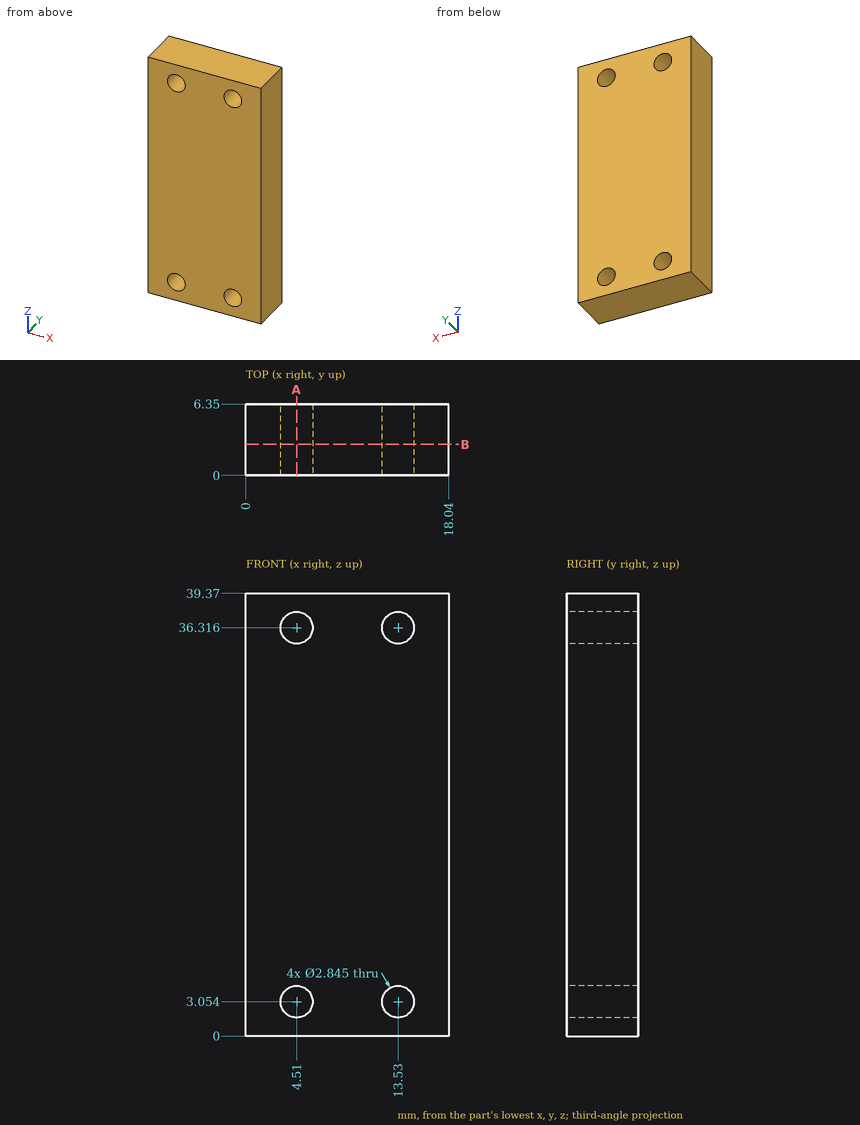
Study the drawing (mm; zero at the part's minimum x, y, z) and answer. Round coordinates to 2 decimals unless told otherwise and drop trailing zeros. Write each loop counter-clockwise with the first axis right and the second up, starting at its lowest first coordinate (ties: lowest second). Pieces come first, ordered by that corner, then holes. Notation, with made-up numbers: (32, 5.5) -> (38, 5.5) arc R17 ccw to (38, 17.5) -> close; hole circle Ø3 at (72.25, 48.5). An arc over 180 degrees is marked (long way). Write item = value, one per line.
1) Section B-B on y = 2.75 is taken. Write down the section's boundary in (x, z) (1 decimal), plus the area to 3 significant figures.
Check values:
outline = (0, 0) -> (18, 0) -> (18, 39.4) -> (0, 39.4) -> close; hole circle Ø2.8 at (4.5, 3.1); hole circle Ø2.8 at (4.5, 36.3); hole circle Ø2.8 at (13.5, 3.1); hole circle Ø2.8 at (13.5, 36.3)
area = 685 mm²
2) Section A-A on x = 4.51 is taken. Write down the section's boundary in (y, z).
Check values:
outline = (0, 0) -> (6.35, 0) -> (6.35, 1.63) -> (0, 1.63) -> close; (0, 4.48) -> (6.35, 4.48) -> (6.35, 34.89) -> (0, 34.89) -> close; (0, 37.74) -> (6.35, 37.74) -> (6.35, 39.37) -> (0, 39.37) -> close
3) Given pin 1 (1.7 mm diameter, centred on x = 13.53, z = 36.32, fed in from -Y), flat-ended and moving along its own axis, determine where the tip first touches the part or whether it passes through.
Check values:
pin_1 = through
4) Straight lines are drawn through the part: line 1 along Z through (x, y) = (13.53, 5.25); line 2 along Z through (x, y) = (3.25, 5.75) (1 decimal); line 3 along X through (y, z) = (5.75, 3.5). For each, find the intervals that lie inside material, in ascending order. Write a range as [from, to].
Check values:
line_1 = [0, 1.63], [4.48, 34.89], [37.74, 39.37]
line_2 = [0, 2.4], [3.7, 35.7], [37, 39.4]
line_3 = [0, 3.16], [5.86, 12.18], [14.88, 18.04]
